The drawing under review shows one solid part. Ordinate dimensions are in mm from its lowest x, y, z. A direction names the side the tool comes from. Give positions to 0.01 mm unless a question says otherwise; leave off trailing zeros. Loops run counter-clockwise (first coordinate to the right, second up) from the corner with the lowest first, then second, coordinate; pieces in that order, holes last. Notation, with made-up numbers: M 29.5,37.5 L 77.5,37.5 A20 ccw 77.5,55.5 Z; hole C 38,-38 d8. An arc over 180 degrees is marked long. Answer as CSV lines item,"result".
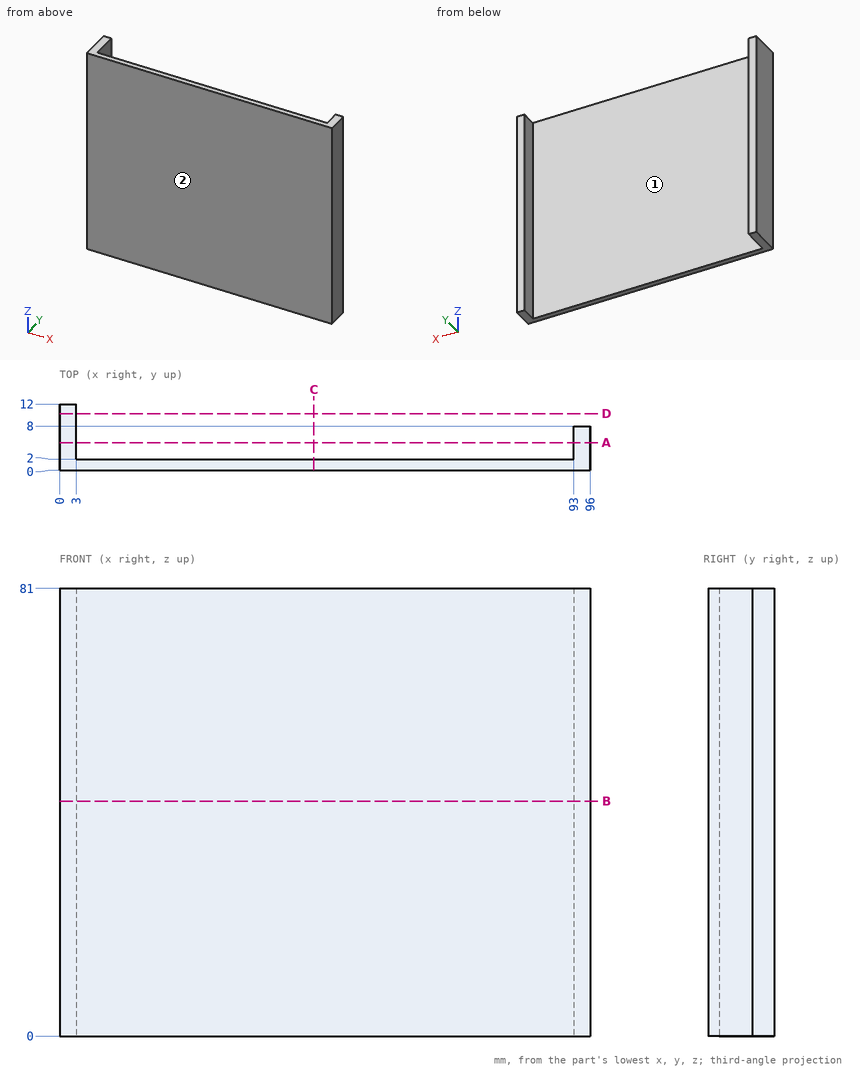
1. We need section D-D, the plane y = 10.25. Write out the cut boundary in (x, z).
Answer block:
outline,"M 0,0 L 3,0 L 3,81 L 0,81 Z"
2. We need section B-B, the plane z = 42.5. Write out the cut boundary in (x, y).
Answer block:
outline,"M 0,0 L 96,0 L 96,8 L 93,8 L 93,2 L 3,2 L 3,12 L 0,12 Z"
3. For the marked faces 1 and 2, list the 3-axis set-ups (+Z, -Z, +X, -X, +Y, -Y) from which the entire face can be reached by the end or side of a thin tool; tool diameter is ignored.
Answer block:
face 1,"+Z, -Z, +Y"
face 2,"+Z, -Z, +X, -X, -Y"
4. We need section C-C, the plane x = 46. Write out the cut boundary in (y, z).
Answer block:
outline,"M 0,0 L 2,0 L 2,81 L 0,81 Z"
5. For P1, Ø24.5, axis at x = 51.5, z = 26, coming from the +Y side; P2, Ø2.5, axis at x = 94.5, z = 40, coming from the +Y side, all flat-tipped, find the tip position at first contact; note any pin that passes through.
Answer block:
P1,"y = 2"
P2,"y = 8"
6. To check wall thickness, follow L1, parallel to X at y = 2.75, z = 9; L2, parallel to Y at x = 77, z = 26; L3, parallel to X at y = 9.25, z = 7. State the ranges of each line that lie inside material, in increasing order. Write a range as [from, to].
Answer block:
L1,"[0, 3], [93, 96]"
L2,"[0, 2]"
L3,"[0, 3]"
7. We need section A-A, the plane y = 5. Write out the cut boundary in (x, z).
Answer block:
outline,"M 0,0 L 3,0 L 3,81 L 0,81 Z; M 93,0 L 96,0 L 96,81 L 93,81 Z"
